The model under review builds one solid part; all positions refer to its coordinate system, in mm. Give positions to 0.01 mm unless a question says otherwise; leave off trailing zeros. Loops run counter-clockwise (first coordinate to the right, second up) from the corner with the lowest first, then second, coordinate; pieces in that order, holes last. Notation, with made-up numbers: (-38.75, -33) - (-33.75, -33) arc R17 cw to (-33.75, -7) - close; hole circle Ø8 at (-38, 49). An arc over 180 degrees is marked (long way). Answer as a JSON object with one key per item and string values.
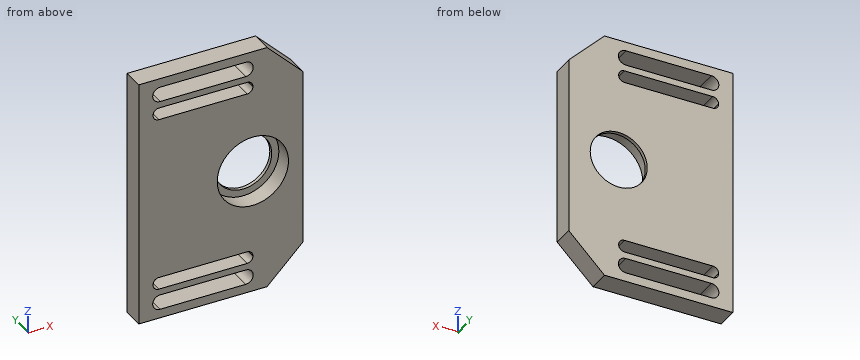
from build123d import *

# Parameters (mm, degrees)
SKIZZE1_W                       = 14
SKIZZE1_H                       = 1.7
AUFSATZ_LINEAR_AUSTRAGEN1_DEPTH = 1.5
VERRUNDUNG1_R                   = 0.8
SKIZZE4_R                       = 5
SCHNITT_LINEAR_AUSTRAGEN1_DEPTH = 2.5
SKIZZE4_3_R                     = 4
SCHNITT_LINEAR_AUSTRAGEN2_DEPTH = 4


with BuildPart() as part:
    # Skizze1 → Aufsatz-Linear austragen1 (new body, symmetric)
    with BuildSketch(Plane(origin=(0, 0, 0), x_dir=(1, 0, 0), z_dir=(0, 1, 0))):
        Polygon((-9, 17.5), (9, 17.5), (14, 12.5), (14, -12.5), (9, -17.5), (-9, -17.5), align=None)
        with BuildLine():
            Line((-6, -16.25), (6, -16.25))
            ThreePointArc((6, -16.25), (7.05, -15.2), (6, -14.15))
            Line((6, -14.15), (-6, -14.15))
            ThreePointArc((-6, -14.15), (-7.05, -15.2), (-6, -16.25))
        make_face(mode=Mode.SUBTRACT)
        with Locations((0, 12.4)):
            Rectangle(SKIZZE1_W, SKIZZE1_H, mode=Mode.SUBTRACT)
        with BuildLine():
            Line((-6, 16.25), (6, 16.25))
            ThreePointArc((6, 16.25), (7.05, 15.2), (6, 14.15))
            Line((6, 14.15), (-6, 14.15))
            ThreePointArc((-6, 14.15), (-7.05, 15.2), (-6, 16.25))
        make_face(mode=Mode.SUBTRACT)
        with Locations((0, -12.4)):
            Rectangle(SKIZZE1_W, SKIZZE1_H, mode=Mode.SUBTRACT)
    extrude(amount=AUFSATZ_LINEAR_AUSTRAGEN1_DEPTH, both=True)

    # Verrundung1
    verrundung1_edges = [part.edges().sort_by_distance(p)[0] for p in [
        (-7, 0, -11.55),
        (-7, 0, -13.25),
        (7, 0, -13.25),
        (7, 0, -11.55),
        (7, 0, 13.25),
        (-7, 0, 13.25),
        (-7, 0, 11.55),
        (7, 0, 11.55),
    ]]
    fillet(verrundung1_edges, radius=VERRUNDUNG1_R)

    # Skizze4 → Schnitt-Linear austragen1 (cut)
    with BuildSketch(Plane.XZ.offset(1.5)):
        with Locations((7, 0)):
            Circle(SKIZZE4_R)
    extrude(amount=-SCHNITT_LINEAR_AUSTRAGEN1_DEPTH, mode=Mode.SUBTRACT)

    # Skizze4<3> → Schnitt-Linear austragen2 (cut, through all)
    with BuildSketch(Plane.XZ.offset(1.5)):
        with Locations((7, 0)):
            Circle(SKIZZE4_3_R)
    extrude(amount=-SCHNITT_LINEAR_AUSTRAGEN2_DEPTH, mode=Mode.SUBTRACT)


solid = part.part
Q1. Consider section B-B, the plane x = 1.25. State the section outline as (y, z) points, plus the area to 3 significant figures.
Results:
{"outline": "(-1.5, -17.5) - (1.5, -17.5) - (1.5, -16.25) - (-1.5, -16.25) - close; (-1.5, -14.15) - (1.5, -14.15) - (1.5, -13.25) - (-1.5, -13.25) - close; (-1.5, -11.55) - (1.5, -11.55) - (1.5, 11.55) - (-1.5, 11.55) - close; (-1.5, 13.25) - (1.5, 13.25) - (1.5, 14.15) - (-1.5, 14.15) - close; (-1.5, 16.25) - (1.5, 16.25) - (1.5, 17.5) - (-1.5, 17.5) - close", "area": "82.2 mm^2"}
Q2. Clearance check with a flat-ended pin moving along its axis: pin 1 Ø11 at (x, z) = (5.5, -1) entering from -Y. State where the tip first meets the part, or that it passes through.
Results:
{"pin 1": "stops at y = -1.5"}
Q3. Consider section D-D, the plane x = 7.75. State the section outline as (y, z) points, plus the area to 3 significant figures.
Results:
{"outline": "(-1.5, -17.5) - (1.5, -17.5) - (1.5, -3.93) - (1, -3.93) - (1, -4.94) - (-1.5, -4.94) - close; (-1.5, 4.94) - (1, 4.94) - (1, 3.93) - (1.5, 3.93) - (1.5, 17.5) - (-1.5, 17.5) - close", "area": "76.4 mm^2"}
Q4. Consider section A-A, the plane z = -15.2. State the section outline as (x, y) points.
Results:
{"outline": "(-9, -1.5) - (-7.05, -1.5) - (-7.05, 1.5) - (-9, 1.5) - close; (7.05, -1.5) - (11.3, -1.5) - (11.3, 1.5) - (7.05, 1.5) - close"}
Q5. To check wall thickness, follow probe 1 along Z at (x, y) = (-4.25, 0.6); probe 2 along Z at (x, y) = (5.75, 0.3); probe 3 along X at (y, z) = (-0.35, -12). State the ranges of each line that lie inside material, in increasing order. Write a range as [from, to].
Results:
{"probe 1": "z = [-17.5, -16.25], [-14.15, -13.25], [-11.55, 11.55], [13.25, 14.15], [16.25, 17.5]", "probe 2": "z = [-17.5, -16.25], [-14.15, -13.25], [-11.55, -4.84], [4.84, 11.55], [13.25, 14.15], [16.25, 17.5]", "probe 3": "x = [-9, -6.92], [6.92, 14]"}
Q6. Consider section C-C, the plane y = -0.6. State how many separate pieces and enclosed holes the cut face has, plus the area to 3 significant figures.
Results:
{"separate pieces": "1", "enclosed holes": "5", "area": "598 mm^2"}
